from build123d import *

# Parameters (mm, degrees)
CYLINDER002_R     = 290
CYLINDER002_DEPTH = 20
CYLINDER001_R     = 296
CYLINDER001_DEPTH = 20
BOX_W             = 290
BOX_H             = 10
BOX_DEPTH         = 10
ARRAY003_COUNT    = 6


with BuildPart() as cilindro002:
    # Cylinder002 → Cylinder002 (new body)
    with BuildSketch(Plane.XY.offset(-535)):
        Circle(CYLINDER002_R)
    extrude(amount=CYLINDER002_DEPTH)


with BuildPart() as cut004:
    # Cylinder001 → Cylinder001 (new body)
    with BuildSketch(Plane.XY.offset(-535)):
        Circle(CYLINDER001_R)
    extrude(amount=CYLINDER001_DEPTH)

    # Cut003: cut Cilindro002
    add(cilindro002.part, mode=Mode.SUBTRACT)


with BuildPart() as fusion015:
    # Box → Box (new body)
    with BuildSketch(Plane(origin=(0, -5, -525), x_dir=(1, 0, 0), z_dir=(0, 0, 1))):
        with Locations((145, 5)):
            Rectangle(BOX_W, BOX_H)
    extrude(amount=BOX_DEPTH)

    # Array003: Fusion015 ×6 about axis
    array003_axis = Axis((0, 0, 0), (0, 0, 1))


with BuildPart() as fusion015_1:
    add(fusion015.part)
    for i in range(1, ARRAY003_COUNT):
        add(fusion015.part.rotate(array003_axis, i * 360 / ARRAY003_COUNT))

    # Fusion013: union Cut004
    add(cut004.part)


solid = fusion015_1.part
Can you work these out from the model? Positions are in its coordinate system, mm. A direction names the side the tool comes from. Round coordinates to 2 decimals unless told otherwise and drop trailing zeros. Order: outer loops, then holes, each group sorted by start corner. A loop starts at its lowest first (then second) coordinate and runs counter-clockwise, first axis right, second up. Notation, with made-up numbers: M 52.5,0 L 89.5,0 A21 ccw 89.5,31 Z; hole C 89.5,20 d9. An arc over 180 degrees is marked long. Use a Markdown table: item, result.
1) If I drill on line 1 along Y through (x, z) = (0, -520.5); line 2 along Y through (x, z) = (86.5, -524.75); line 3 along Y through (x, z) = (166.5, -516), over which ranges is the centre line in solid material (lowest first)?
Geometry says:
| item | result |
|---|---|
| line 1 | y = -296 to -290, -10 to 10, 290 to 296 |
| line 2 | y = -283.08 to -276.8, -159.82 to -139.82, -5 to 5, 139.82 to 159.82, 276.8 to 283.08 |
| line 3 | y = -244.73 to -237.44, -5 to 5, 237.44 to 244.73 |
2) Imagine slicing it at A-A (x = 243). List the corners of the cut face in (y, z) for me, then the cut area to 3 significant figures.
Geometry says:
| item | result |
|---|---|
| outline | M -169.02,-535 L -158.28,-535 L -158.28,-515 L -169.02,-515 Z; M -5,-525 L 5,-525 L 5,-515 L -5,-515 Z; M 158.28,-535 L 169.02,-535 L 169.02,-515 L 158.28,-515 Z |
| area | 530 mm² |
3) On a 3-axis mill with a long thin cutter (end or side, diameter ignored), from which of +Z, -Z, +X, -X, +Y, -Y can I reach the whole of each face in a straight line? I mean faces 1 (the face through (-78, 125.1, -520.1)), 2 (the face through (-1, 1, -515)), 3 (the face through (-1, 1, -525)). Say none if no direction works.
Geometry says:
| item | result |
|---|---|
| face 1 | +Z, -Z |
| face 2 | +Z, +X, -X, +Y, -Y |
| face 3 | -Z |
4) Imagine slicing it at B-B (y = 108). List the corners of the cut face in (x, z) for me.
Geometry says:
| item | result |
|---|---|
| outline | M -275.59,-535 L -269.14,-535 L -269.14,-515 L -275.59,-515 Z; M -68.13,-525 L -56.58,-525 L -56.58,-515 L -68.13,-515 Z; M 56.58,-525 L 68.13,-525 L 68.13,-515 L 56.58,-515 Z; M 269.14,-535 L 275.59,-535 L 275.59,-515 L 269.14,-515 Z |
5) If we mould it in two halves opening along X, with no side actions, what happens to faces 4 (the face through (196, -218, -535)), 5 (the face through (-69.34, -130.1, -520.07)), 6 (the face through (-64, -289, -525))? For each: +X half, -X half, draft (parallel to the pull), parting line (faces both ways), or undercut.
Geometry says:
| item | result |
|---|---|
| face 4 | draft |
| face 5 | undercut |
| face 6 | parting line |
6) I'm going to push flat-ended pins straight in: P1, Ø1.5, axis at y = 157, z = -532.5, coming from the +X side; P2, Ø1, axis at y = -201, z = -517.5, coming from the +X side; P3, Ø11, axis at x = -161.5, z = -517.5, coming from the -Y side. Where does each tip first touch, or does it pass through?
Geometry says:
| item | result |
|---|---|
| P1 | stops at x = 251.4 |
| P2 | stops at x = 217.75 |
| P3 | stops at y = -251.56 |
7) Imagine slicing it at D-D (x = 95). List the corners of the cut face in (y, z) for me.
Geometry says:
| item | result |
|---|---|
| outline | M -280.34,-535 L -274,-535 L -274,-515 L -280.34,-515 Z; M -174.54,-525 L -154.54,-525 L -154.54,-515 L -174.54,-515 Z; M -5,-525 L 5,-525 L 5,-515 L -5,-515 Z; M 154.54,-525 L 174.54,-525 L 174.54,-515 L 154.54,-515 Z; M 274,-535 L 280.34,-535 L 280.34,-515 L 274,-515 Z |
8) Imagine slicing it at C-C (z = -521). List the corners of the cut face in (x, y) for me, then the cut area to 3 significant figures.
Geometry says:
| item | result |
|---|---|
| outline | C 0,0 d592; hole M -289.96,-5 A290 ccw -149.31,-248.61 L -8.66,-5 Z; hole M -289.96,5 L -8.66,5 L -149.31,248.61 A290 ccw Z; hole M -140.65,-253.61 A290 ccw 140.65,-253.61 L 0,-10 Z; hole M -140.65,253.61 L 0,10 L 140.65,253.61 A290 ccw Z; hole M 8.66,-5 L 149.31,-248.61 A290 ccw 289.96,-5 Z; hole M 8.66,5 L 289.96,5 A290 ccw 149.31,248.61 Z |
| area | 28,200 mm² |
